Read the model definition and answer for the solid it produces. Units are mm, in the model's axes. A direction names the side the tool comes from. Give positions to 0.01 mm unless a question says otherwise; leave off trailing zeros. Write each loop counter-clockwise with the first axis right and the second up, starting at its lowest first coordinate (ties: lowest second). Pieces come first, ordered by that corner, then holes.
Autodesk Inventor part; units mm, degrees
ref_plane "YZ Plane" through (0, 0, 0) normal (1, 0, 0) x (0, 1, 0)
ref_plane "XZ Plane" through (0, 0, 0) normal (0, 1, 0) x (-1, 0, 0)
ref_plane "XY Plane" through (0, 0, 0) normal (0, 0, 1) x (1, 0, 0)
sketch "Boceto1" plane through (0, 0, 0) normal (0, 0, 1) x (1, 0, 0)
  line L0 (-25, 22.5) -> (25, 22.5)
  line L1 (30, 17.5) -> (30, -17.5)
  line L2 (25, -22.5) -> (-25, -22.5)
  line L3 (-30, -17.5) -> (-30, 17.5)
  line L4 (-30, 22.5) -> (30, -22.5) construction
  line L5 (30, 22.5) -> (-30, -22.5) construction
  line L6 (-25, 20.5) -> (25, 20.5)
  line L7 (28, 17.5) -> (28, -17.5)
  line L8 (25, -20.5) -> (-25, -20.5)
  line L9 (-28, -17.5) -> (-28, 17.5)
  arc A0 (-30, -17.5) -> (-25, -22.5) centre (-25, -17.5) ccw
  arc A1 (25, -22.5) -> (30, -17.5) centre (25, -17.5) ccw
  arc A2 (30, 17.5) -> (25, 22.5) centre (25, 17.5) ccw
  arc A3 (-25, 22.5) -> (-30, 17.5) centre (-25, 17.5) ccw
  arc A4 (-25, 20.5) -> (-28, 17.5) centre (-25, 17.5) ccw
  arc A5 (28, 17.5) -> (25, 20.5) centre (25, 17.5) ccw
  arc A6 (25, -20.5) -> (28, -17.5) centre (25, -17.5) ccw
  arc A7 (-28, -17.5) -> (-25, -20.5) centre (-25, -17.5) ccw
  point P0 (0, 0)
  point P1 (-28, 20.5)
  point P2 (28, 20.5)
  point P3 (28, -20.5)
  point P4 (-28, -20.5)
  dimension "d0" = 45
  dimension "d1" = 2
  dimension "d5" = 5
  dimension "d6" = 3
extrude "Extrusión1" add sketch "Boceto1" along normal blind 10 contours L0 A2 L1 A1 L2 A0 L3 A3 | L6 A5 L7 A6 L8 A7 L9 A4
shell "Vaciado1" thickness 1 removed faces 1 at (-8.3333, -7.5, 0)
sketch "Boceto2" plane through (0, 0, 0) normal (0, 0, -1) x (-1, 0, 0)
  line L0 (25, -22.5) -> (-25, -22.5)
  arc A0 (-30, -17.5) -> (-25, -22.5) centre (-25, -17.5) ccw
  line L1 (-30, -17.5) -> (-30, 17.5)
  arc A1 (-25, 22.5) -> (-30, 17.5) centre (-25, 17.5) ccw
  line L2 (-25, 22.5) -> (25, 22.5)
  arc A2 (30, 17.5) -> (25, 22.5) centre (25, 17.5) ccw
  line L3 (30, 17.5) -> (30, -17.5)
  arc A3 (25, -22.5) -> (30, -17.5) centre (25, -17.5) ccw
  line L4 (30, 0) -> (40, 0)
  line L5 (-30, 0) -> (-40, 0)
  circle A4 centre (35, 0) radius 5
  circle A5 centre (-35, 0) radius 5
  circle A6 centre (35, 0) radius 2.1
  circle A7 centre (-35, 0) radius 2.1
  circle A8 centre (37.5, -12.2474) radius 7.5
  line L6 (30, 17.5) -> (30, -17.5)
  circle A9 centre (-37.5, 12.2474) radius 7.5
  circle A10 centre (-37.5, -12.2474) radius 7.5
  circle A11 centre (37.5, 12.2474) radius 7.5
  line L7 (-30, -17.5) -> (-30, 17.5)
  point P0 (0, 0)
  point P1 (-36, -4.899)
  point P2 (-30, -12.2474)
  point P3 (-30, 12.2474)
  point P4 (-36, 4.899)
  point P5 (36, 4.899)
  point P6 (30, 12.2474)
  point P7 (30, -12.2474)
  point P8 (36, -4.899)
  dimension "d8" = 10
  dimension "d9" = 10
  dimension "d10" = 4.2
  dimension "d11" = 4.2
  dimension "d12" = 15
  dimension "d14" = 15
  dimension "d15" = 15
  dimension "d16" = 15
extrude "Extrusión2" add sketch "Boceto2" against normal blind 10 contours L3 A4 A8 | A10 A5 L1 | A4 L4 A6 | L3 A11 A4 | L4 A6 A4 | A5 A9 L1 | A5 L5 A7 | L5 A7 A5 | A6 L4 | L4 A6 | A7 L5 | L5 A7
sketch "Boceto3" plane through (0, 0, 0) normal (0, 0, -1) x (-1, 0, 0)
  arc A0 (-36, 4.899) -> (-36, -4.899) centre (-35, 0) ccw
  arc A1 (36, -4.899) -> (36, 4.899) centre (35, 0) ccw
  point P0 (0, 0)
hole "Agujero1" at (35, 0, 0) at (-35, 0, 0) direction (0, 0, 1) diameter 4.2 depth 5
properties part number "Deshumidicador"
Item 1: Which of the six approach directions +Z, -Z, +X, -X, +Y, -Y give full straight-line access (tool end or side, diameter ignored) to faces 4 (the flat face through (29, 0, 4)), 5 (the flat face through (30, -15, 5)), 6 (the cylindrical face through (-40, 0, 5))?
Result set:
face 4: -Z
face 5: +Z, -Z, +X, -Y
face 6: +Z, -Z, -X
Item 2: Section D-D (x = 2) is taken. Write down the section's boundary in (y, z), and give its area (3 significant figures).
Result set:
outline: (-22.5, 0) - (-21.5, 0) - (-21.5, 9) - (21.5, 9) - (21.5, 0) - (22.5, 0) - (22.5, 10) - (-22.5, 10) - close
area: 63.0 mm2
Item 3: Section B-B (z = 2.25) is taken. Write down the section's boundary in (x, y).
Result set:
outline: (-36, -4.9) arc R7.5 cw to (-30, -12.25) - (-30, -17.5) arc R5 ccw to (-25, -22.5) - (25, -22.5) arc R5 ccw to (30, -17.5) - (30, -12.25) arc R7.5 cw to (36, -4.9) arc R5 ccw to (36, 4.9) arc R7.5 cw to (30, 12.25) - (30, 17.5) arc R5 ccw to (25, 22.5) - (-25, 22.5) arc R5 ccw to (-30, 17.5) - (-30, 12.25) arc R7.5 cw to (-36, 4.9) arc R5 ccw to start; hole circle Ø4.2 at (-35, 0); hole (-29, -17.5) arc R4 ccw to (-25, -21.5) - (25, -21.5) arc R4 ccw to (29, -17.5) - (29, 17.5) arc R4 ccw to (25, 21.5) - (-25, 21.5) arc R4 ccw to (-29, 17.5) - close; hole circle Ø4.2 at (35, 0)
Item 4: Section C-C (z = 6.75) is taken. Write down the section's boundary in (x, y), and give its area (3 significant figures).
Result set:
outline: (-36, -4.9) arc R7.5 cw to (-30, -12.25) - (-30, -17.5) arc R5 ccw to (-25, -22.5) - (25, -22.5) arc R5 ccw to (30, -17.5) - (30, -12.25) arc R7.5 cw to (36, -4.9) arc R5 ccw to (36, 4.9) arc R7.5 cw to (30, 12.25) - (30, 17.5) arc R5 ccw to (25, 22.5) - (-25, 22.5) arc R5 ccw to (-30, 17.5) - (-30, 12.25) arc R7.5 cw to (-36, 4.9) arc R5 ccw to start; hole (-29, -17.5) arc R4 ccw to (-25, -21.5) - (25, -21.5) arc R4 ccw to (29, -17.5) - (29, 17.5) arc R4 ccw to (25, 21.5) - (-25, 21.5) arc R4 ccw to (-29, 17.5) - close
area: 419 mm2
Item 5: Section A-A (y = -14.5) is taken. Write down the section's boundary in (x, z).
Result set:
outline: (-30, 0) - (-29, 0) - (-29, 9) - (29, 9) - (29, 0) - (30, 0) - (30, 10) - (-30, 10) - close
Item 6: Find the intervals of material crossed by line 1 along X through (y, z) = (0, 1.65); line 2 along X through (y, z) = (14, 7.5); line 3 along Y through (x, z) = (-16, 5.5), in increasing order.
Result set:
line 1: x = -40 to -37.1, -32.9 to -29, 29 to 32.9, 37.1 to 40
line 2: x = -30 to -29, 29 to 30
line 3: y = -22.5 to -21.5, 21.5 to 22.5
Item 7: Each of these flat-tipped pins is pushed along its axis until it touches: pin 1 Ø2.5 at (y, z) = (-14.5, 4) entering from -X; pin 2 Ø10 at (x, y) = (-8.5, -15) entering from -Z; pin 3 Ø2.5 at (y, z) = (-1, 4) entering from +X; pin 4 Ø6 at (y, z) = (16, 5) entering from +X. Where does it stop, or does it pass through?
Result set:
pin 1: stops at x = -30
pin 2: stops at z = 9
pin 3: stops at x = 40
pin 4: stops at x = 30
Item 8: Determine the mould class of faces 1 (the flat face through (0, 21.5, 4)), 2 (the cylindrical face through (-28.57, 21, 4.93)), 3 (the flat face through (30, 15, 5)) for opening direction X: pulls with the +X half, pulls with the -X half, needs draft (parallel to the pull), parting line crosses it, or undercut.
Result set:
face 1: undercut
face 2: pulls with the -X half
face 3: pulls with the +X half
